from build123d import *

# Parameters (mm, degrees)
BOSS_EXTRU_1_DEPTH      = 8
ESQUISSE3_W             = 2.1
ESQUISSE3_H             = 3.5
ENL_V_MAT_EXTRU_1_DEPTH = 3
ESQUISSE4_OUTSIDE_W     = 15.69
ESQUISSE4_OUTSIDE_H     = 11.69
ESQUISSE4_OUTSIDE_W_2   = 5.1
ESQUISSE4_OUTSIDE_H_2   = 6.7
ENL_V_MAT_EXTRU_2_DEPTH = 3
CONG_1_R                = 0.5
CHANFREIN1_SIZE         = 0.4
CHANFREIN1_SIZE2        = 0.857802768


with BuildPart() as part:
    # Esquisse2 → Boss.-Extru.1 (new body)
    with BuildSketch(Plane.XY):
        with BuildLine():
            Line((1.1, 0), (9.6, 0))
            ThreePointArc((9.6, 0), (10.377817459, 0.322182541), (10.7, 1.1))
            Line((10.7, 1.1), (10.7, 5.6))
            ThreePointArc((10.7, 5.6), (10.377817459, 6.377817459), (9.6, 6.7))
            Line((9.6, 6.7), (1.1, 6.7))
            ThreePointArc((1.1, 6.7), (0.322182541, 6.377817459), (0, 5.6))
            Line((0, 5.6), (0, 1.1))
            ThreePointArc((0, 1.1), (0.322182541, 0.322182541), (1.1, 0))
        make_face()
    extrude(amount=BOSS_EXTRU_1_DEPTH)

    # Esquisse3 → Enlèv. mat.-Extru.1 (cut)
    with BuildSketch(Plane.XY.offset(8)):
        with Locations((5.2, 3.5)):
            Rectangle(ESQUISSE3_W, ESQUISSE3_H)
    extrude(amount=-ENL_V_MAT_EXTRU_1_DEPTH, mode=Mode.SUBTRACT)

    # Esquisse4 outside → Enlèv. mat.-Extru.2 (cut)
    with BuildSketch(Plane.XY.offset(8)):
        with Locations((5.35, 3.35)):
            Rectangle(ESQUISSE4_OUTSIDE_W, ESQUISSE4_OUTSIDE_H)
        with Locations((5.2, 3.35)):
            Rectangle(ESQUISSE4_OUTSIDE_W_2, ESQUISSE4_OUTSIDE_H_2, mode=Mode.SUBTRACT)
    extrude(amount=-ENL_V_MAT_EXTRU_2_DEPTH, mode=Mode.SUBTRACT)

    # Congé1
    cong_1_edges = [part.edges().sort_by_distance(p)[0] for p in [
        (5.2, 6.7, 8),
        (5.2, 0, 8),
        (10.7, 3.35, 5),
        (1.875, 6.7, 5),
        (0.322182541, 6.377817459, 5),
        (0, 3.35, 5),
        (0.322182541, 0.322182541, 5),
        (1.875, 0, 5),
        (8.675, 0, 5),
        (10.377817459, 0.322182541, 5),
        (10.377817459, 6.377817459, 5),
        (8.675, 6.7, 5),
        (7.75, 6.7, 6.5),
        (7.75, 3.35, 8),
        (7.75, 0, 6.5),
        (2.65, 0, 6.5),
        (2.65, 3.35, 8),
        (2.65, 6.7, 6.5),
    ]]
    fillet(cong_1_edges, radius=CONG_1_R)

    # Chanfrein1
    chanfrein1_edges = [part.edges().sort_by_distance(p)[0] for p in [
        (5.35, 6.7, 0),
        (10.377817459, 6.377817459, 0),
        (10.7, 3.35, 0),
        (10.377817459, 0.322182541, 0),
        (5.35, 0, 0),
        (0.322182541, 0.322182541, 0),
        (0, 3.35, 0),
        (0.322182541, 6.377817459, 0),
    ]]
    chanfrein1_side = [part.faces().sort_by_distance(p)[0] for p in [
        (5.35, 3.35, 0),
    ]]
    chamfer(chanfrein1_edges, length=CHANFREIN1_SIZE, length2=CHANFREIN1_SIZE2, reference=chanfrein1_side[0])


solid = part.part
The listing builds one solid part. Answer for the finished solid, in the listing's coordinates (mm). A direction names the side the tool comes from. Round coordinates to 2 decimals unless told otherwise and drop trailing zeros. Order: outer loops, then holes, each group sorted by start corner. A loop starts at its lowest first (then second) coordinate and runs counter-clockwise, first axis right, second up. Notation, with made-up numbers: (29.25, 14.25) -> (57.25, 14.25) arc R21 ccw to (57.25, 30.25) -> close; hole circle Ø11 at (49.5, 76.5). An arc over 180 degrees is marked (long way). Put each result on its own line as item: value.
Q1. Each of these flat-tipped pins is pushed along its axis until it touches: P1, Ø2, axis at x = 9.5, y = 2.5, coming from the +Z side; P2, Ø2.5, axis at y = 4, z = 6, coming from the +X side; P3, Ø1, axis at y = 4.5, z = 6.5, coming from the +X side; P4, Ø2.5, axis at x = 5, y = 4, coming from the +Z side. Where does it stop, or does it pass through?
Results list:
P1: z = 5
P2: x = 10.63
P3: x = 7.75
P4: z = 8
Q2. Determine the mould class of faces 1 (the flat face through (7.75, 3, 6)), 2 (the flat face through (5, 3, 0)), 3 (the flat face through (6.25, 3, 7)) for opening direction X: pulls with the +X half, pulls with the -X half, needs draft (parallel to the pull), parting line crosses it, or undercut.
Results list:
face 1: pulls with the +X half
face 2: needs draft
face 3: undercut
Q3. Consider line 1 along X through (y, z) = (3, 6.5); line 2 along X through (y, z) = (6.25, 6); line 3 along Z through (x, y) = (2, 3.25). Determine where each line is inside the solid, lowest interval first.
Results list:
line 1: 2.65 to 4.15, 6.25 to 7.75
line 2: 2.65 to 7.75
line 3: 0 to 5
Q4. Which of the six approach directions +Z, -Z, +X, -X, +Y, -Y give full straight-line access (tool end or side, diameter ignored) to faces 4 (the cylindrical face through (0.331, 6.386, 2.653)), 5 (the flat face through (2.65, 3, 6)), 6 (the flat face through (5, 4, 5))?
Results list:
face 4: +Z, -Z, -X, +Y
face 5: +Z, -X, +Y, -Y
face 6: +Z
Q5. Section A-A, the plane z = 6.75 is taken. Write down the section's boundary in (x, y), and give its area (3 significant figures).
Results list:
outline: (2.65, 0.5) arc R0.5 ccw to (3.15, 0) -> (7.25, 0) arc R0.5 ccw to (7.75, 0.5) -> (7.75, 6.2) arc R0.5 ccw to (7.25, 6.7) -> (3.15, 6.7) arc R0.5 ccw to (2.65, 6.2) -> close; hole (4.15, 1.75) -> (6.25, 1.75) -> (6.25, 5.25) -> (4.15, 5.25) -> close
area: 26.6 mm^2
Q6. Section C-C, the plane x = 5 is taken. Write down the section's boundary in (y, z), and give its area (3 significant figures).
Results list:
outline: (0, 0.86) -> (0.4, 0) -> (6.3, 0) -> (6.7, 0.86) -> (6.7, 7.5) arc R0.5 ccw to (6.2, 8) -> (5.25, 8) -> (5.25, 5) -> (1.75, 5) -> (1.75, 8) -> (0.5, 8) arc R0.5 ccw to (0, 7.5) -> close
area: 42.6 mm^2
Q7. Section B-B, the plane y = 1.25 is taken. Write down the section's boundary in (x, z).
Results list:
outline: (0, 0.86) -> (0.4, 0) -> (10.3, 0) -> (10.7, 0.86) -> (10.7, 4.5) arc R0.5 ccw to (10.2, 5) -> (7.75, 5) -> (7.75, 7.5) arc R0.5 ccw to (7.25, 8) -> (3.15, 8) arc R0.5 ccw to (2.65, 7.5) -> (2.65, 5) -> (0.5, 5) arc R0.5 ccw to (0, 4.5) -> close
Q8. Section D-D, the plane x = 1.5 is taken. Write down the section's boundary in (y, z).
Results list:
outline: (0, 0.86) -> (0.4, 0) -> (6.3, 0) -> (6.7, 0.86) -> (6.7, 4.5) arc R0.5 ccw to (6.2, 5) -> (0.5, 5) arc R0.5 ccw to (0, 4.5) -> close
